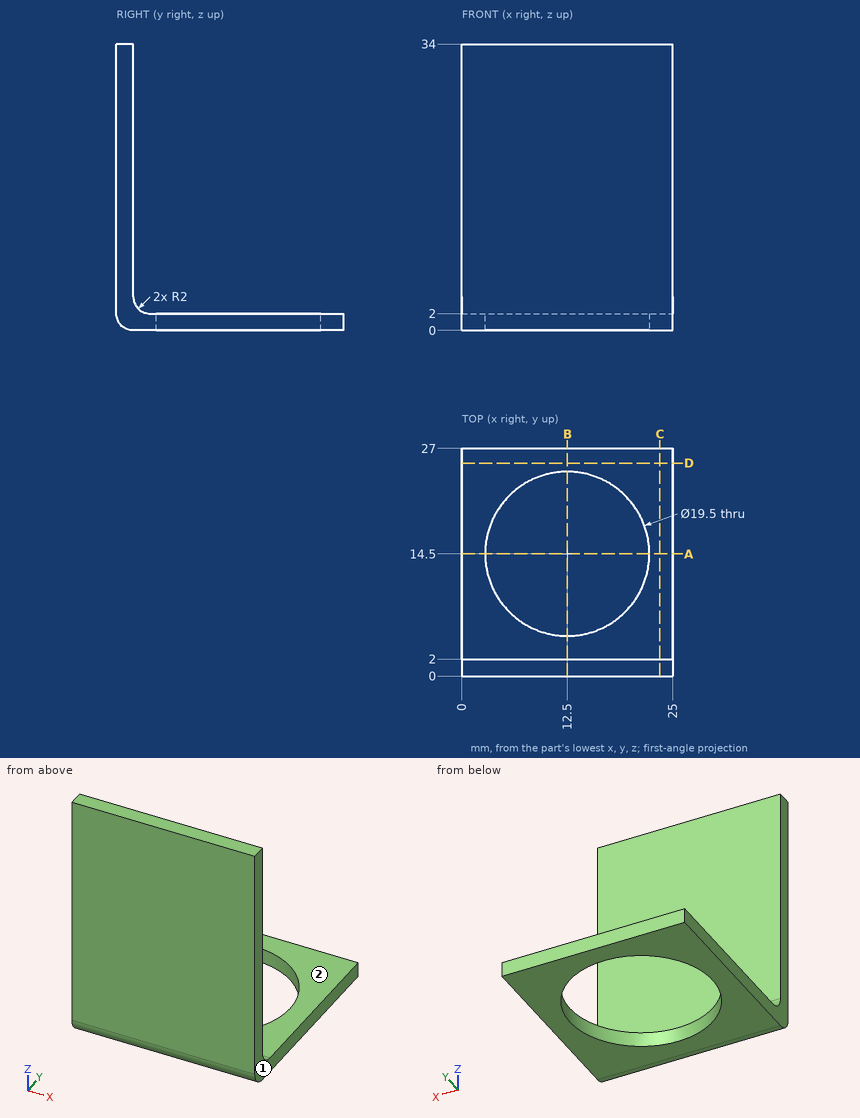
Geometry check sheet. Reference: drawing and pictorial views, mm from the part's lowest x, y, z. A direction names the side the tool comes from. Round coordinates to 2 decimals unless told otherwise and drop trailing zeros. Loops run counter-clockwise (first coordinate to the right, second up) from the corner with the lowest first, then second, coordinate; pieces in that order, holes last. Notation, with made-up numbers: M 45,34 L 59,34 A14 ccw 59,44 Z; hole C 14,8.25 d5. An arc over 180 degrees is marked long. Return JSON: item names as keys, results as strings. Group by question number.
(1) Section check D-D, the plane y = 25.25. Enter the section's corners in (x, z).
(2) Scan lines: line 1 along Y through (x, z) = (5, 14.5); line 2 along Y through (x, z) = (12.5, 0.8). Record each from-to range of solid material in increasing order. Write a range as [from, to].
(3) Set-up check for the marked faces 1 and 2: record each of +Z, -Z, +X, -X, +Y, -Y from which the full face is reachable in a straight line by a thin tool's end or side.
(4) Section check A-A, the plane y = 14.5. Enter the section's corners in (x, z).
(5) Section check B-B, the plane x = 12.5. Enter the section's corners in (y, z), and give its area (3 significant figures).
(6) Go/stop test with a flat-tipped pin: pin 1 (6 mm diameter, centred on x = 10, y = 21.5, fed in from +Z). Record where the tip stops, or that it passes through.
(7) Section check C-C, the plane x = 23.5. Enter the section's corners in (y, z), and give its area (3 significant figures).
Data:
{
 "1": {"outline": "M 0,0 L 25,0 L 25,2 L 0,2 Z"},
 "2": {"line 1": "[0, 2]", "line 2": "[0.4, 4.75], [24.25, 27]"},
 "3": {"face 1": "+Z, -Z, +X, +Y, -Y", "face 2": "+Z, +X, -X, +Y"},
 "4": {"outline": "M 0,0 L 2.75,0 L 2.75,2 L 0,2 Z; M 22.25,0 L 25,0 L 25,2 L 22.25,2 Z"},
 "5": {"outline": "M 0,2 A2 ccw 2,0 L 4.75,0 L 4.75,2 L 4,2 A2 cw 2,4 L 2,34 L 0,34 Z; M 24.25,0 L 27,0 L 27,2 L 24.25,2 Z", "area": "79.0 mm²"},
 "6": {"pin 1": "z = 2"},
 "7": {"outline": "M 0,2 A2 ccw 2,0 L 27,0 L 27,2 L 4,2 A2 cw 2,4 L 2,34 L 0,34 Z", "area": "118 mm²"}
}
